```python
from build123d import *

# Parameters (mm, degrees)
F1_DEPTH = 6.35
F3_D     = 6.858
F3_DEPTH = 12.7
F5_DEPTH = 25.4


with BuildPart() as f1:
    # F0 (on Front) → F1 (new body)
    with BuildSketch(Plane.XZ):
        with BuildLine():
            ThreePointArc((0, 49.53), (-3.367596, 48.135096), (-4.7625, 44.7675))
            Line((-4.7625, 44.7675), (-4.7625, 4.7625))
            ThreePointArc((-4.7625, 4.7625), (-3.367596, 1.394904), (0, 0))
            Line((0, 0), (39.0525, 0))
            Line((39.0525, 0), (39.0525, 3.175))
            Line((39.0525, 3.175), (39.0525, 14.2875))
            Line((39.0525, 14.2875), (39.0525, 35.2425))
            Line((39.0525, 35.2425), (39.0525, 46.355))
            Line((39.0525, 46.355), (39.0525, 49.53))
            Line((39.0525, 49.53), (0, 49.53))
        make_face()
    extrude(amount=F1_DEPTH)

    # F3
    with Locations(Plane.XZ.offset(6.35)):
        with Locations((17.145, 24.765)):
            Hole(F3_D / 2, depth=F3_DEPTH)

    # F4 (on face) → F5 (cut)
    with BuildSketch(Plane(origin=(0, 0, 0), x_dir=(-1, 0, 0), z_dir=(0, 1, 0))):
        with BuildLine():
            ThreePointArc((-20.955, 43.02125), (-19.271202, 42.323798), (-18.57375, 40.64))
            ThreePointArc((-18.57375, 40.64), (-19.271202, 38.956202), (-20.955, 38.25875))
            Line((-20.955, 38.25875), (-13.335, 38.25875))
            ThreePointArc((-13.335, 38.25875), (-15.71625, 40.64), (-13.335, 43.02125))
            Line((-13.335, 43.02125), (-20.955, 43.02125))
        make_face()
        with BuildLine():
            ThreePointArc((-20.955, 38.25875), (-19.271202, 38.956202), (-18.57375, 40.64))
            ThreePointArc((-18.57375, 40.64), (-19.271202, 42.323798), (-20.955, 43.02125))
            ThreePointArc((-20.955, 43.02125), (-23.33625, 40.64), (-20.955, 38.25875))
        make_face()
        with BuildLine():
            ThreePointArc((-10.95375, 40.64), (-11.651202, 42.323798), (-13.335, 43.02125))
            ThreePointArc((-13.335, 43.02125), (-15.71625, 40.64), (-13.335, 38.25875))
            ThreePointArc((-13.335, 38.25875), (-11.651202, 38.956202), (-10.95375, 40.64))
        make_face()
    extrude(amount=-F5_DEPTH, mode=Mode.SUBTRACT)


solid = f1.part
```
Geometry check sheet. Reference: the model listing, model coordinates, mm. A direction names the side the tool comes from. Coordinates: 2 decimals unless noted, no trailing zeros. Order: outer loops, then holes, each group sorted by start corner. A loop starts at its lowest first (then second) coordinate and runs counter-clockwise, first axis right, second up. Notation, with made-up numbers: (29.5, 78.5) - (69.5, 78.5) arc R5 cw to (69.5, 85.5) - close; hole circle Ø10 at (-29.75, 64.25). An arc over 180 degrees is marked (long way). Answer as a JSON object with one key per item and string values. Group by question number.
Item 1: Sectioned sample at A-A, the plane y = -5. Record the cut outline in (x, z) (1 decimal).
Item 2: Draft check along X on faces 1 (the face through (17, -3, 38.259)), 2 (the face through (17, -6.35, 20)), 3 (the face through (-3.3, -3.1, 48.2)). Enter one of: +X half, -X half, draft (parallel to the pull), parting line (faces both ways), or undercut.
Item 3: Sectioned sample at B-B, the plane x = 15.5. Record the cut outline in (y, z).
Item 4: Tool access check on faces 4 (the face through (23.336, -3.131, 40.692)), 5 (the face through (-4.762, -3, 25)). Record the directions out of +Z, -Z, +X, -X, +Y, -Y that give a thin tool (end or side, any length) a straight path to the whole face; none if there is none.
Item 5: Scan lines: probe 1 along X at (y, z) = (-4.5, 24.5); probe 2 along Z at (x, y) = (13.5, -1); probe 3 along Z at (x, y) = (15.5, -2). Record each from-to range of solid material in increasing order.
Resolved:
{
 "1": {"outline": "(-4.8, 4.8) arc R4.8 ccw to (0, 0) - (39.1, 0) - (39.1, 49.5) - (0, 49.5) arc R4.8 ccw to (-4.8, 44.8) - close; hole (13.3, 38.3) - (21, 38.3) arc R2.4 ccw to (21, 43) - (13.3, 43) arc R2.4 ccw to start; hole circle Ø6.9 at (17.1, 24.8)"},
 "2": {"face 1": "undercut", "face 2": "draft", "face 3": "-X half"},
 "3": {"outline": "(-6.35, 0) - (0, 0) - (0, 21.76) - (-6.35, 21.76) - close; (-6.35, 27.77) - (0, 27.77) - (0, 38.26) - (-6.35, 38.26) - close; (-6.35, 43.02) - (0, 43.02) - (0, 49.53) - (-6.35, 49.53) - close"},
 "4": {"face 4": "+Y, -Y", "face 5": "+Z, -Z, -X, +Y, -Y"},
 "5": {"probe 1": "-4.76 to 13.73, 20.56 to 39.05", "probe 2": "0 to 38.26, 43.02 to 49.53", "probe 3": "0 to 21.76, 27.77 to 38.26, 43.02 to 49.53"}
}
